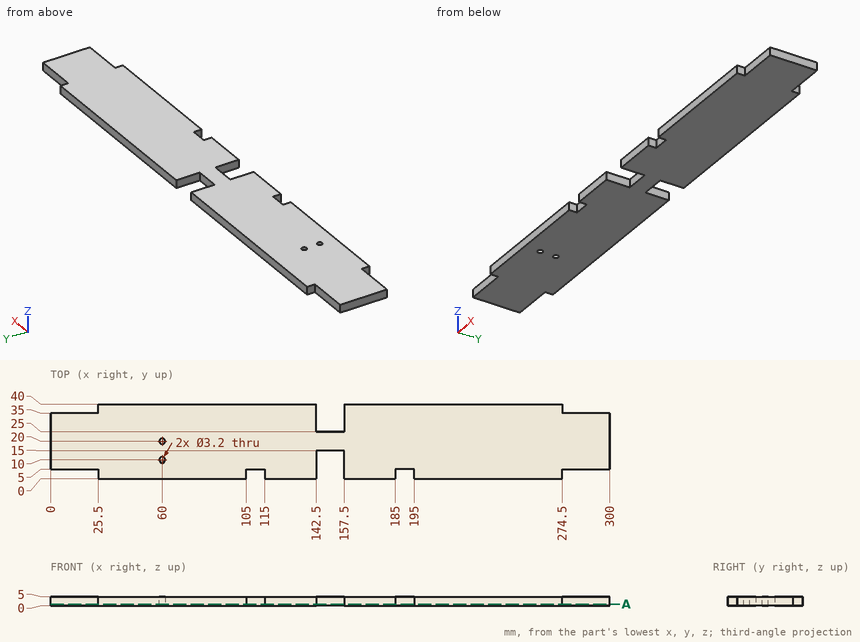
The drawing under review shows one solid part. Ordinate dimensions are in mm from its lowest x, y, z. Coordinates: 2 decimals unless noted, no trailing zeros. Answer in a Markdown table with one row per item. Add a question column.
Q1. For probe 1 along Y at (x, z) = (60, 1.5); probe 2 along X at (y, z) = (2.5, 0.95); probe 3 along X at (y, z) = (38, 3), list the stretches that pass through material, from the lowest coordinate up.
Q2. For P1, Ø2.5, axis at x = 149.5, z = 2, coming from the +Y side; P2, Ø2.5, axis at y = 3.5, z = 1.5, coming from the -X side; P3, Ø2.5, axis at x = 16, z = 1.5, coming from the +Y side; P4, Ø1, axis at x = 118, z = 2.5, coming from the -Y side, all flat-tipped, find the tip position at first contact; note any pin that passes through.
Q3. We need section A-A, the plane z = 1. Count the separate pieces of the cut face and the enclosed holes in it, and give its area (3 significant figures).
Answer list:
| question | item | result |
|---|---|---|
| 1 | probe 1 | y = 0 to 8.4, 11.6 to 18.4, 21.6 to 40 |
| 1 | probe 2 | x = 25.5 to 105, 115 to 142.5, 157.5 to 185, 195 to 274.5 |
| 1 | probe 3 | x = 25.5 to 142.5, 157.5 to 274.5 |
| 2 | P1 | stops at y = 25 |
| 2 | P2 | stops at x = 25.5 |
| 2 | P3 | stops at y = 35 |
| 2 | P4 | stops at y = 0 |
| 3 | separate pieces | 1 |
| 3 | enclosed holes | 2 |
| 3 | area | 10,900 mm2 |
